```python
from build123d import *

# Parameters (mm, degrees)
SKETCH2_R           = 2.5796875
BOSS_EXTRUDE1_DEPTH = 1.27


with BuildPart() as part:
    # Sketch2 → Boss-Extrude1 (new body)
    with BuildSketch(Plane.XY):
        with BuildLine():
            ThreePointArc((0, 22.225), (7.9375, 30.1625), (15.875, 22.225))
            Line((15.875, 22.225), (15.875, 0))
            Line((15.875, 0), (0, 0))
            Line((0, 0), (0, 22.225))
        make_face()
        with Locations((7.9375, 22.225)):
            Circle(SKETCH2_R, mode=Mode.SUBTRACT)
    extrude(amount=BOSS_EXTRUDE1_DEPTH)


solid = part.part
```
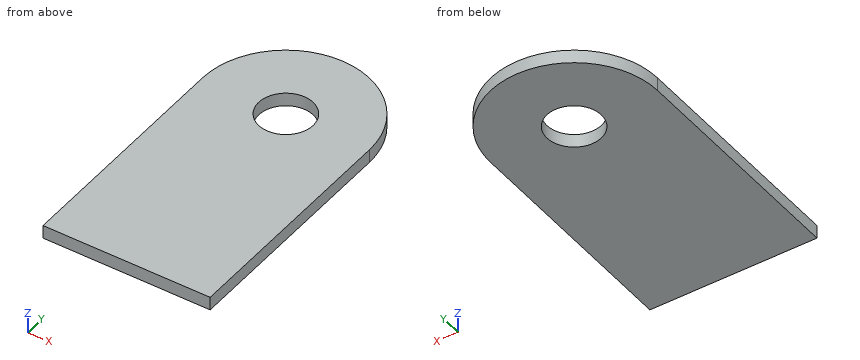
Here's how the part is built. I have some questions about the finished solid (model axes, mm). Round coordinates to 2 decimals unless told otherwise and drop trailing zeros. Write each loop counter-clockwise with the first axis right and the second up, starting at its lowest first coordinate (ties: lowest second). Pieces come first, ordered by that corner, then holes. Notation, with made-up numbers: M -33,-6 L 1,-6 A25 ccw 1,30 Z; hole C 30,67.25 d3. An arc over 180 degrees is marked long. Answer as CSV lines item,"result". Start each with the question number.
1. Suppose I cut it at A-A on z = 0.6. Write out the boundary of the cut face in (x, y) (1 decimal), then the cut area to 3 significant figures.
2. Suppose I cut it at C-C on x = 7. Write out the boundary of the cut face in (y, z), then the cut area to 3 significant figures.
3. Suppose I cut it at B-B on y = 23. Write out the boundary of the cut face in (x, z).
4. I need wall thicknesses on probe 1 along Y at (x, z) = (9.25, 0.4); probe 2 along Y at (x, z) = (6, 0.65); probe 3 along Y at (x, z) = (14.75, 0.7). Which ranges of each line are inside material? Lowest first, please.
5. Suppose I cut it at D-D on x = 3. Write out the boundary of the cut face in (y, z), then the cut area to 3 significant figures.
Check result:
1,outline,"M 0,0 L 15.9,0 L 15.9,22.2 A7.9 ccw 0,22.2 Z; hole C 7.9,22.2 d5.2"
1,area,"431 mm2"
2,outline,"M 0,0 L 19.82,0 L 19.82,1.27 L 0,1.27 Z; M 24.63,0 L 30.11,0 L 30.11,1.27 L 24.63,1.27 Z"
2,area,"32.1 mm2"
3,outline,"M 0.04,0 L 5.48,0 L 5.48,1.27 L 0.04,1.27 Z; M 10.4,0 L 15.84,0 L 15.84,1.27 L 10.4,1.27 Z"
4,probe 1,"y = 0 to 20, 24.45 to 30.05"
4,probe 2,"y = 0 to 20.52, 23.93 to 29.92"
4,probe 3,"y = 0 to 26.3"
5,outline,"M 0,0 L 28.44,0 L 28.44,1.27 L 0,1.27 Z"
5,area,"36.1 mm2"
